from build123d import *

# Parameters (mm, degrees)
PAD_DEPTH       = 6.5
POCKET_DEPTH    = 6
SKETCH002_R     = 13.5
POCKET001_DEPTH = 1
SKETCH003_W     = 5.4
SKETCH003_H     = 6.5
PAD001_DEPTH    = 3.8
POCKET002_DEPTH = 10
SKETCH008_R     = 0.6
POCKET003_DEPTH = 2
SKETCH009_R     = 0.6
POCKET004_DEPTH = 2
FILLET_R        = 2.9
FILLET001_R     = 2.9
FILLET002_R     = 5
FILLET003_R     = 5
FILLET004_R     = 5
FILLET005_R     = 5
SKETCH010_W     = 3.95
SKETCH010_H     = 6.5
PAD002_DEPTH    = 4.5
POCKET005_DEPTH = 10
SKETCH012_R     = 0.6
POCKET006_DEPTH = 2
SKETCH013_R     = 0.6
POCKET007_DEPTH = 2
FILLET006_R     = 3.4
FILLET007_R     = 3.4
SKETCH014_R     = 20.45
SKETCH014_R_2   = 19.5
POCKET008_DEPTH = 0.3
SKETCH015_R     = 0.9
PAD003_DEPTH    = 6
FILLET008_R     = 1
POCKET009_DEPTH = 4
POCKET010_DEPTH = 4


with BuildPart() as part:
    # Sketch → Pad (new body)
    with BuildSketch(Plane.XY):
        with BuildLine():
            Line((-22.5019915649, 16), (-22.5019915649, -16))
            Line((-22.5019915649, -16), (-16.2858834578, -17.9))
            ThreePointArc((-16.2858834578, -17.9), (0.2206895736, -24.1989937004), (16.6096357576, -17.6))
            Line((16.6096357576, -17.6), (25.6083856708, -17.45))
            Line((25.6083856708, 17.45), (25.6083856708, -17.45))
            Line((16.6096357576, 17.6), (25.6083856708, 17.45))
            ThreePointArc((16.6096357576, 17.6), (0.2206895736, 24.1989937004), (-16.2858834578, 17.9))
            Line((-22.5019915649, 16), (-16.2858834578, 17.9))
        make_face()
    extrude(amount=PAD_DEPTH)

    # Sketch001 → Pocket (cut)
    with BuildSketch(Plane.XY):
        with BuildLine():
            Line((-14.8539557021, 16.9), (-21.2122180433, 15.55))
            Line((-21.2122180433, 15.55), (-21.2122180433, -15.55))
            Line((-21.2122180433, -15.55), (-14.8539557021, -16.9))
            ThreePointArc((-14.8539557021, -16.9), (-0.0760301383, -22.4998715423), (14.739402973, -17))
            Line((14.739402973, -17), (23.6191552218, -16.4))
            Line((23.6191552218, 16.4), (23.6191552218, -16.4))
            Line((14.739402973, 17), (23.6191552218, 16.4))
            ThreePointArc((14.739402973, 17), (-0.0760301383, 22.4998715423), (-14.8539557021, 16.9))
        make_face()
    extrude(amount=POCKET_DEPTH, mode=Mode.SUBTRACT)

    # Sketch002 (on Face19 of Pocket) → Pocket001 (cut)
    with BuildSketch(Plane(origin=(0, 0, 6), x_dir=(1, 0, 0), z_dir=(0, 0, -1))):
        Circle(SKETCH002_R)
    extrude(amount=-POCKET001_DEPTH, mode=Mode.SUBTRACT)

    # Sketch003 (on Face6 of Pocket001) → Pad001 (join)
    with BuildSketch(Plane.YZ.offset(25.6083856708)):
        with Locations((-14.75, 3.25)):
            Rectangle(SKETCH003_W, SKETCH003_H)
        with Locations((14.75, 3.25)):
            Rectangle(SKETCH003_W, SKETCH003_H)
    extrude(amount=PAD001_DEPTH)

    # Sketch006 → Pocket002 (cut)
    with BuildSketch(Plane.XY.offset(6.5)):
        with BuildLine():
            ThreePointArc((25.6083856708, 17.45), (27.3544703324, 16.0634214301), (29.4083856708, 15.1957558499))
            Line((29.4083856708, 17.45), (29.4083856708, 15.1957558499))
            Line((29.4083856708, 17.45), (25.6083856708, 17.45))
        make_face()
        with BuildLine():
            ThreePointArc((29.4083856708, -15.1957558499), (27.3544703324, -16.0634214301), (25.6083856708, -17.45))
            Line((29.4083856708, -17.45), (25.6083856708, -17.45))
            Line((29.4083856708, -15.1957558499), (29.4083856708, -17.45))
        make_face()
    extrude(amount=-POCKET002_DEPTH, mode=Mode.SUBTRACT)

    # Sketch008 (on Face27 of Pocket002) → Pocket003 (cut)
    with BuildSketch(Plane(origin=(0, -12.05, 0), x_dir=(-1, 0, 0), z_dir=(0, 1, 0))):
        with Locations((-27.7083856708, 1.7)):
            Circle(SKETCH008_R)
    extrude(amount=-POCKET003_DEPTH, mode=Mode.SUBTRACT)

    # Sketch009 (on Face26 of Pocket003) → Pocket004 (cut)
    with BuildSketch(Plane.XZ.offset(-12.05)):
        with Locations((27.7083856708, 1.7)):
            Circle(SKETCH009_R)
    extrude(amount=-POCKET004_DEPTH, mode=Mode.SUBTRACT)

    # Fillet
    fillet_edges = [part.edges().sort_by_distance(p)[0] for p in [
        (29.408386, -13.622878, 6.5),
    ]]
    fillet(fillet_edges, radius=FILLET_R)

    # Fillet001
    fillet001_edges = [part.edges().sort_by_distance(p)[0] for p in [
        (29.408386, 13.622878, 6.5),
    ]]
    fillet(fillet001_edges, radius=FILLET001_R)

    # Fillet002
    fillet002_edges = [part.edges().sort_by_distance(p)[0] for p in [
        (16.609636, -17.6, 3.25),
    ]]
    fillet(fillet002_edges, radius=FILLET002_R)

    # Fillet003
    fillet003_edges = [part.edges().sort_by_distance(p)[0] for p in [
        (16.609636, 17.6, 3.25),
    ]]
    fillet(fillet003_edges, radius=FILLET003_R)

    # Fillet004
    fillet004_edges = [part.edges().sort_by_distance(p)[0] for p in [
        (-16.285883, -17.9, 3.25),
    ]]
    fillet(fillet004_edges, radius=FILLET004_R)

    # Fillet005
    fillet005_edges = [part.edges().sort_by_distance(p)[0] for p in [
        (-16.285883, 17.9, 3.25),
    ]]
    fillet(fillet005_edges, radius=FILLET005_R)

    # Sketch010 (on Face4 of Fillet005) → Pad002 (join)
    with BuildSketch(Plane(origin=(-22.5019915649, 0, 0), x_dir=(0, -1, 0), z_dir=(-1, 0, 0))):
        with Locations((-14.025, 3.25)):
            Rectangle(SKETCH010_W, SKETCH010_H)
        with Locations((14.025, 3.25)):
            Rectangle(SKETCH010_W, SKETCH010_H)
    extrude(amount=PAD002_DEPTH)

    # Sketch011 (on Face6 of Pad002) → Pocket005 (cut)
    with BuildSketch(Plane.XY.offset(6.5)):
        with BuildLine():
            ThreePointArc((-27.0019915649, 14.6), (-24.6759937451, 15.0557212933), (-22.5019915649, 16))
            Line((-22.5019915649, 16), (-27.0019915649, 16))
            Line((-27.0019915649, 16), (-27.0019915649, 14.6))
        make_face()
        with BuildLine():
            ThreePointArc((-22.5019915649, -16), (-24.6759937451, -15.0557212933), (-27.0019915649, -14.6))
            Line((-27.0019915649, -14.6), (-27.0019915649, -16))
            Line((-27.0019915649, -16), (-22.5019915649, -16))
        make_face()
    extrude(amount=-POCKET005_DEPTH, mode=Mode.SUBTRACT)

    # Sketch012 (on Face23 of Pocket005) → Pocket006 (cut)
    with BuildSketch(Plane(origin=(0, -12.05, 0), x_dir=(-1, 0, 0), z_dir=(0, 1, 0))):
        with Locations((25.3019915649, 1.7)):
            Circle(SKETCH012_R)
    extrude(amount=-POCKET006_DEPTH, mode=Mode.SUBTRACT)

    # Sketch013 (on Face21 of Pocket006) → Pocket007 (cut)
    with BuildSketch(Plane.XZ.offset(-12.05)):
        with Locations((-25.3019915649, 1.7)):
            Circle(SKETCH013_R)
    extrude(amount=-POCKET007_DEPTH, mode=Mode.SUBTRACT)

    # Fillet006
    fillet006_edges = [part.edges().sort_by_distance(p)[0] for p in [
        (-27.001992, 13.325, 6.5),
    ]]
    fillet(fillet006_edges, radius=FILLET006_R)

    # Fillet007
    fillet007_edges = [part.edges().sort_by_distance(p)[0] for p in [
        (-27.001992, -13.325, 6.5),
    ]]
    fillet(fillet007_edges, radius=FILLET007_R)

    # Sketch014 (on Face4 of Fillet007) → Pocket008 (cut)
    with BuildSketch(Plane.XY.offset(6.5)):
        Circle(SKETCH014_R)
        Circle(SKETCH014_R_2, mode=Mode.SUBTRACT)
    extrude(amount=-POCKET008_DEPTH, mode=Mode.SUBTRACT)

    # Sketch015 (on Face55 of Pocket008) → Pad003 (join)
    with BuildSketch(Plane(origin=(0, 0, 6), x_dir=(1, 0, 0), z_dir=(0, 0, -1))):
        with Locations((-18.42, 13.32)):
            Circle(SKETCH015_R)
        with Locations((-18.42, -13.32)):
            Circle(SKETCH015_R)
        with Locations((7.27, 18.56)):
            Circle(SKETCH015_R)
        with Locations((5.37, -19.79)):
            Circle(SKETCH015_R)
    extrude(amount=PAD003_DEPTH)

    # Fillet008
    fillet008_edges = [part.edges().sort_by_distance(p)[0] for p in [
        (-19.32, -13.32, 6),
        (6.37, -18.56, 6),
        (-19.32, 13.32, 6),
        (4.47, 19.79, 6),
    ]]
    fillet(fillet008_edges, radius=FILLET008_R)

    # Sketch016 (on Face16 of Fillet008) → Pocket009 (cut)
    with BuildSketch(Plane(origin=(0, 0, 0), x_dir=(1, 0, 0), z_dir=(0, 0, -1))):
        with BuildLine():
            Line((-5, 23.6778377391), (-5, 21.9374109685))
            ThreePointArc((5, 21.9374109685), (0, 22.5), (-5, 21.9374109685))
            Line((5, 23.6778377391), (5, 21.9374109685))
            ThreePointArc((5, 23.6778377391), (0, 24.2), (-5, 23.6778377391))
        make_face()
    extrude(amount=-POCKET009_DEPTH, mode=Mode.SUBTRACT)

    # Sketch017 → Pocket010 (cut)
    with BuildSketch(Plane.XY):
        with BuildLine():
            Line((-3.499984119, -22.2261132717), (-3.5, -23.9455632634))
            ThreePointArc((-3.5, -23.9455632634), (0, -24.2000019575), (3.5, -23.9455632634))
            Line((3.5000158811, -22.2261082701), (3.5, -23.9455632634))
            ThreePointArc((-3.499984119, -22.2261132717), (1.60767e-05, -22.5), (3.5000158811, -22.2261082701))
        make_face()
        with BuildLine():
            ThreePointArc((-13.9498796389, -17.6536358312), (-11.25, -19.4855715851), (-8.3135572795, -20.9077680626))
            Line((-8.3135572795, -20.9077680626), (-8.9416927184, -22.487466094))
            ThreePointArc((-15.0038705449, -18.987466094), (-12.1, -20.9578147716), (-8.9416927184, -22.487466094))
            Line((-13.9498796389, -17.6536358312), (-15.0038705449, -18.987466094))
        make_face()
        with BuildLine():
            ThreePointArc((8.3135572795, -20.9077680626), (11.25, -19.4855715851), (13.9498796389, -17.6536358312))
            Line((13.9498796389, -17.6536358312), (15.0038705449, -18.987466094))
            ThreePointArc((8.9416927184, -22.487466094), (12.1, -20.9578147716), (15.0038705449, -18.987466094))
            Line((8.3135572795, -20.9077680626), (8.9416927184, -22.487466094))
        make_face()
    extrude(amount=POCKET010_DEPTH, mode=Mode.SUBTRACT)


solid = part.part
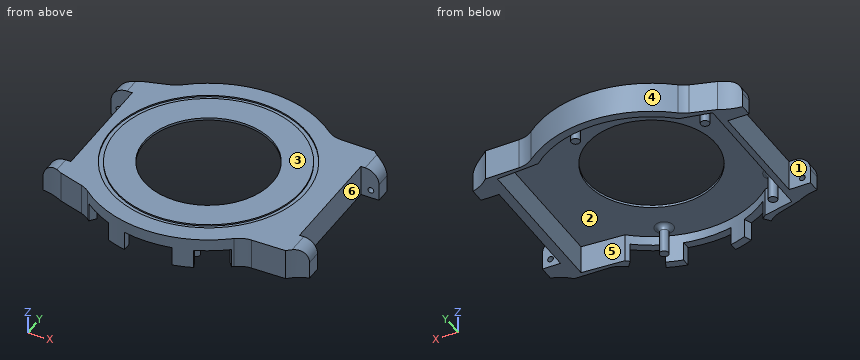
Verification items for the finished model (mm, model axes). Face numbers are marked on the shaded views. A direction names the side the tool comes from. Coordinates: 2 decimals unless noted, no trailing zeros. Order: outer loops, then holes, each group sorted by start corner. A loop starts at its lowest first (then second) coordinate and runs counter-clockwise, first axis right, second up. Notation, with made-up numbers: M 30.5,33 L 74.5,33 A15 cw 74.5,61 Z; hole C 33,-0.75 d10. An arc over 180 degrees is marked long. One line per item, written item: value. Start each with the question number.
Item 1: Sectioned sample at B-B (x = 10). Enter the section's corners in (y, z).
Item 2: Access from +Z, -Z, +X, -X, +Y, -Y to the whole of each face (thin tool, end or side, straight path). Record for the marked faces 1, 2 and 3.
Item 3: Scan lines: probe 1 along Y at (x, z) = (0, 6.1); probe 2 along X at (y, z) = (-1, 2.5); probe 3 along Y at (x, z) = (-18, 4.5). Record each from-to range of solid material in increasing order.
Item 4: Sectioned sample at C-C (x = 17). Enter the section's corners in (y, z).
Item 5: Gauge pin test, flat ends, axial feed: pin 1 (1 mm diameter, centred on x = -25, z = 1.5, fed in from -Y); pin 2 (0.6 mm diameter, centred on x = 27.5, z = 1.5, fed in from +Y); pin 3 (1.5 mm diameter, centred on y = -0.5, z = 5.5, fed in from +X); pin 4 (1.5 mm diameter, centred on x = 7, y = -11, fed in from +Z). Record the tip position at first contact, or that the pin passes through.
Item 6: Sectioned sample at D-D (x = -18.42). Enter the section's corners in (y, z).
Item 7: Mould release check, pull along X, two halves, no side actions. Record for the marked faces 4, 5 and 6: released by +X, released by -X, zero draft, split by the parting line, or undercut.
Item 8: Sectioned sample at A-A (y = 5). Enter the section's corners in (x, z).
Conclusion:
1. outline: M -22.04,4 L -20.16,4 L -20.16,6 L -9.07,6 L -9.07,6.5 L -16.74,6.5 L -16.74,6.2 L -17.84,6.2 L -17.84,6.5 L -22.04,6.5 Z; M 9.07,6 L 20.16,6 L 20.16,0 L 22.04,0 L 22.04,6.5 L 17.84,6.5 L 17.84,6.2 L 16.74,6.2 L 16.74,6.5 L 9.07,6.5 Z
2. face 1: +Z, -Z, -X
2. face 2: -Z
2. face 3: +Z, +X, -X, +Y, -Y
3. probe 1: y = -24.2 to -13.5, 13.5 to 24.2
3. probe 2: x = -22.5 to -21.21, 23.62 to 25.61
3. probe 3: y = -17.38 to -16.23, -14.12 to -12.52, 12.52 to 14.12, 16.23 to 17.38
4. outline: M -17.81,0 L -16.85,0 L -16.85,6 L 16.85,6 L 16.85,0 L 17.81,0 L 17.81,6.5 L 11.37,6.5 L 11.37,6.2 L 9.55,6.2 L 9.55,6.5 L -9.55,6.5 L -9.55,6.2 L -11.37,6.2 L -11.37,6.5 L -17.81,6.5 Z
5. pin 1: stops at y = -15.11
5. pin 2: stops at y = 16.16
5. pin 3: stops at x = 25.61
5. pin 4: stops at z = 6.5
6. outline: M -17.25,0 L -16.14,0 L -16.14,6 L -15.22,6 A1 cw -14.22,5 L -14.22,0 L -12.42,0 L -12.42,5 A1 cw -11.42,6 L 11.42,6 A1 cw 12.42,5 L 12.42,0 L 14.22,0 L 14.22,5 A1 cw 15.22,6 L 16.14,6 L 16.14,0 L 17.25,0 L 17.25,6.5 L 8.88,6.5 L 8.88,6.2 L 6.4,6.2 L 6.4,6.5 L -6.4,6.5 L -6.4,6.2 L -8.88,6.2 L -8.88,6.5 L -17.25,6.5 Z
7. face 4: split by the parting line
7. face 5: undercut
7. face 6: released by +X
8. outline: M -22.5,0 L -21.21,0 L -21.21,6 L -12.54,6 L -12.54,6.5 L -18.85,6.5 L -18.85,6.2 L -19.83,6.2 L -19.83,6.5 L -22.5,6.5 Z; M 12.54,6 L 23.62,6 L 23.62,0 L 25.61,0 L 25.61,6.5 L 19.83,6.5 L 19.83,6.2 L 18.85,6.2 L 18.85,6.5 L 12.54,6.5 Z
